Read the model definition and answer for the solid it produces. Units are mm, in the model's axes. Face numbers are marked on the shaded views. Coordinates: 2 decimals unless noted, no trailing zeros. Write each loop counter-clockwise with the first axis right and the second up, starting at its lowest first coordinate (ties: lowest second). Pieces come first, ordered by that corner, then holes.
(1) Find the intervals of material crossed by probe 1 along Y at (x, z) = (0, 2.85) (3 decimals); probe 2 along Y at (x, z) = (12, 1.9) (3 decimals); probe 3 along X at (y, z) = (22.5, 1.75), in increasing order.
(2) The mould has two halves that part along X. Classify the marked faces 1, 2 and 3: +X half, -X half, draft (parallel to the pull), parting line (faces both ways), or undercut.
(3) Section A-A on y = -8 is taken. Write down the section's boundary in (x, z).
(4) Section B-B on x = -3.5 is taken. Write down the section's boundary in (y, z), then the cut area to 3 significant figures.
(5) Section D-D on x = 12.5 is taken. Write down the section's boundary in (y, z), then the cut area to 3 significant figures.
(6) Given pin 1 (1 mm diameter, centred on y = 17.5, z = 1.5, fed in from -X); pin 2 (2 mm diameter, centred on y = 19.5, z = 0.5, fed in from -X); pin 3 (1.2 mm diameter, centred on y = -33, z = 1.5, fed in from -X), each flat-ended and moving along its own axis, determine where each tip first touches the part or whether it passes through.
(7) Section C-C on y = -34.5 is taken. Write down the section's boundary in (x, z) (3 decimals).
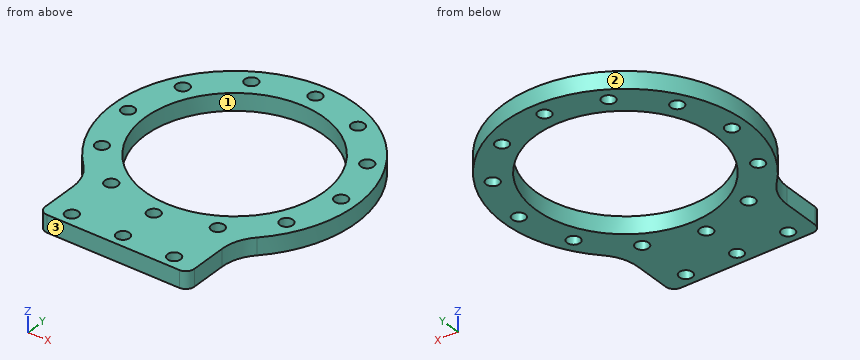
from build123d import *

# Parameters (mm, degrees)
SKETCH_2_R          = 1.525
EXTRUDE_1_DEPTH     = 4
SKETCH_4_R          = 21
CUT_EXTRUDE_1_DEPTH = 5
SKETCH_5_R          = 1.525
CUT_EXTRUDE_2_DEPTH = 5
FILLET_1_R          = 2
FILLET_2_R          = 10


with BuildPart() as part:
    # 草图2 → 凸台-拉伸1 (new body)
    with BuildSketch(Plane.XY):
        with BuildLine():
            ThreePointArc((17.5, -22.494443758), (0, 28.5), (-17.5, -22.494443758))
            Line((-17.5, -22.494443758), (-17.5, -37.5))
            Line((-17.5, -37.5), (17.5, -37.5))
            Line((17.5, -37.5), (17.5, -22.494443758))
        make_face()
        with Locations((-12.5, -21.650635095)):
            Circle(SKETCH_2_R, mode=Mode.SUBTRACT)
        with Locations((12.5, -21.650635095)):
            Circle(SKETCH_2_R, mode=Mode.SUBTRACT)
        with Locations((-21.650635095, -12.5)):
            Circle(SKETCH_2_R, mode=Mode.SUBTRACT)
        with Locations((21.650635095, -12.5)):
            Circle(SKETCH_2_R, mode=Mode.SUBTRACT)
        with Locations((-25, 0)):
            Circle(SKETCH_2_R, mode=Mode.SUBTRACT)
        with Locations((-21.650635095, 12.5)):
            Circle(SKETCH_2_R, mode=Mode.SUBTRACT)
        with Locations((-12.5, 21.650635095)):
            Circle(SKETCH_2_R, mode=Mode.SUBTRACT)
        with Locations((25, 0)):
            Circle(SKETCH_2_R, mode=Mode.SUBTRACT)
        with Locations((0, 25)):
            Circle(SKETCH_2_R, mode=Mode.SUBTRACT)
        with Locations((12.5, 21.650635095)):
            Circle(SKETCH_2_R, mode=Mode.SUBTRACT)
        with Locations((21.650635095, 12.5)):
            Circle(SKETCH_2_R, mode=Mode.SUBTRACT)
        with Locations((0, -25)):
            Circle(SKETCH_2_R, mode=Mode.SUBTRACT)
    extrude(amount=EXTRUDE_1_DEPTH)

    # 草图4 → 切除-拉伸1 (cut, through all)
    with BuildSketch(Plane.XY.offset(4)):
        Circle(SKETCH_4_R)
    extrude(amount=-CUT_EXTRUDE_1_DEPTH, mode=Mode.SUBTRACT)

    # 草图5 → 切除-拉伸2 (cut, through all)
    with BuildSketch(Plane.XY.offset(4)):
        with Locations((0, -34.5)):
            Circle(SKETCH_5_R)
        with Locations((12, -34.5)):
            Circle(SKETCH_5_R)
        with Locations((-12, -34.5)):
            Circle(SKETCH_5_R)
    extrude(amount=-CUT_EXTRUDE_2_DEPTH, mode=Mode.SUBTRACT)

    # 圆角1
    fillet_1_edges = [part.edges().sort_by_distance(p)[0] for p in [
        (17.5, -37.5, 2),
        (-17.5, -37.5, 2),
    ]]
    fillet(fillet_1_edges, radius=FILLET_1_R)

    # 圆角2
    fillet_2_edges = [part.edges().sort_by_distance(p)[0] for p in [
        (17.5, -22.494443758, 2),
        (-17.5, -22.494443758, 2),
    ]]
    fillet(fillet_2_edges, radius=FILLET_2_R)


solid = part.part
Response:
1. probe 1: y = -37.5 to -36.025, -32.975 to -26.525, -23.475 to -21, 21 to 23.475, 26.525 to 28.5
1. probe 2: y = -37.5 to -36.025, -32.975 to -23.091, -20.21 to -17.234, 17.234 to 20.21, 23.091 to 25.851
1. probe 3: x = -17.49 to -13.77, -11.23 to 11.23, 13.77 to 17.49
2. face 1: undercut
2. face 2: parting line
2. face 3: draft
3. outline: (-27.35, 0) - (-19.42, 0) - (-19.42, 4) - (-27.35, 4) - close; (19.42, 0) - (27.35, 0) - (27.35, 4) - (19.42, 4) - close
4. outline: (-37.5, 0) - (-20.71, 0) - (-20.71, 4) - (-37.5, 4) - close; (20.71, 0) - (28.28, 0) - (28.28, 4) - (20.71, 4) - close
4. area: 97.5 mm2
5. outline: (-37.5, 0) - (-35.94, 0) - (-35.94, 4) - (-37.5, 4) - close; (-33.06, 0) - (-23.18, 0) - (-23.18, 4) - (-33.06, 4) - close; (-20.13, 0) - (-16.87, 0) - (-16.87, 4) - (-20.13, 4) - close; (16.87, 0) - (20.13, 0) - (20.13, 4) - (16.87, 4) - close; (23.18, 0) - (25.61, 0) - (25.61, 4) - (23.18, 4) - close
5. area: 81.5 mm2
6. pin 1: stops at x = -22.87
6. pin 2: stops at x = -21.68
6. pin 3: stops at x = -17.5
7. outline: (-17.5, 0) - (-13.525, 0) - (-13.525, 4) - (-17.5, 4) - close; (-10.475, 0) - (-1.525, 0) - (-1.525, 4) - (-10.475, 4) - close; (1.525, 0) - (10.475, 0) - (10.475, 4) - (1.525, 4) - close; (13.525, 0) - (17.5, 0) - (17.5, 4) - (13.525, 4) - close
